Autodesk Inventor part; units mm, degrees
ref_plane "Work Plane1" through (0, 0, 3.175) normal (0, 0, 1) x (1, 0, 0)
ref_plane "YZ Plane" through (0, 0, 0) normal (1, 0, 0) x (0, 1, 0)
ref_plane "XZ Plane" through (0, 0, 0) normal (0, 1, 0) x (-1, 0, 0)
sketch "Sketch1" plane through (0, 0, 0) normal (0, 1, 0) x (-1, 0, 0)
  circle A0 centre (0, 0) radius 3.175
  circle A1 centre (0, 0) radius 1.5
  dimension "d0" = 6.35
  dimension "d1" = 3
extrude "Extrusion1" add sketch "Sketch1" against normal blind 7.5 contours A0 | A1
ref_plane "Work Plane1" through (0, 0, 3.175) normal (0, 0, 1) x (1, 0, 0)
sketch "Sketch2" plane through (0, 0, 3.175) normal (0, 0, 1) x (1, 0, 0)
  line L0 (-3.175, -7.5) -> (3.175, -7.5)
  line L1 (3.175, 0) -> (-3.175, 0)
  line L2 (-3.175, 0) -> (-3.175, -7.5)
  line L3 (-3.175, -2) -> (3.175, -2) construction
  circle A0 centre (0, -4.75) radius 1.5
  dimension "d11" = 2
  dimension "d12" = 3
  dimension "d13" = 2.75
  dimension "d14" = 3.175
hole "Threaded Hole" at (0, -4.75, 3.175) direction (0, 0, -1) diameter 2.459 end through all
hole "Pin Bearing Hole" at (0, 0, 0) direction (0, -1, 0) diameter 3.2004 depth 4.75 tip angle 118
equation "\"d9\" = d11 + d13"
properties part number "Bearing Nut" material "Steel, Alloy"
Input: part model. Units: mm. Frame: model coordinates. Round coordinates to 2 decimals unless told otherwise and drop trailing zeros. Order: outer loops, then holes, each group sorted by start corner. A loop starts at its lowest first (then second) coordinate and runs counter-clockwise, first axis right, second up. Notation, with made-up numbers: (75.5, -1) - (80.5, -1) arc R10 ccw to (80.5, 6) - close; hole circle Ø2 at (-8.5, -24.75). An arc over 180 degrees is marked (long way). Answer as a JSON object with one key per item and string values. Group by question number.
(1) Material intervals for probe 1 along Y at (x, z) = (0, -0.5); probe 2 along X at (y, z) = (-5.5, -0.5); probe 3 along X at (y, z) = (-4.75, 1.25), sorted ascending. Write a range as from..to.
(2) Pin query (flat end, axial travel): P1, Ø2, axis at y = -3.5, z = -1.5, coming from the -X side; P2, Ø1, axis at y = -3.5, z = -1.5, coming from the -X side. Return the tip coordinate at first contact, or that it passes through.
(3) Cut plane B-B (y = -4.25). Return loops of the section in (x, z) (3 decimals).
(4) Cut plane A-A (x = 0). Return loops of the section in (y, z) (1 decimal), then the cut area to 3 significant figures.
(5) Cut plane D-D (y = -2.25). Return loops of the section in (x, z) (3 decimals), then the cut area to 3 significant figures.
(6) Draft query along X for faces 1 (the face through (0, -7.5, 0)), 2 (the face through (0.471, -5.886, -0.044)), 3 (the face through (-1.5, -3.7, -2.8)), 4 (the face through (-0.07, -2.41, -1.6)). Return one class per face: released by +X, released by -X, zero draft, split by the parting line, or undercut.
Here are the results:
{
 "1": {"probe 1": "y = -7.5..-5.98", "probe 2": "x = -3.14..-0.97, 0.97..3.14", "probe 3": "x = -2.92..-1.23, 1.23..2.92"},
 "2": {"P1": "stops at x = -3.14", "P2": "stops at x = -3.01"},
 "3": {"outline": "(-1.123, -2.97) - (-1.123, -1.14) arc R1.6 cw to (-1.123, 1.14) - (-1.123, 2.97) arc R3.175 ccw to start; (1.123, -2.97) arc R3.175 ccw to (1.123, 2.97) - (1.123, 1.14) arc R1.6 cw to (1.123, -1.14) - close"},
 "4": {"outline": "(-7.5, -3.2) - (-6, -3.2) - (-6, 3.2) - (-7.5, 3.2) - close; (-3.5, -3.2) - (0, -3.2) - (0, -1.6) - (-3.5, -1.6) - close; (-3.5, 1.6) - (0, 1.6) - (0, 3.2) - (-3.5, 3.2) - close", "area": "20.7 mm^2"},
 "5": {"outline": "circle Ø6.35 at (0, 0); hole circle Ø3.2 at (0, 0)", "area": "23.6 mm^2"},
 "6": {"face 1": "zero draft", "face 2": "undercut", "face 3": "split by the parting line", "face 4": "undercut"}
}
